from build123d import *

# Parameters (mm, degrees)
SKIZZE1_W                                            = 38
SKIZZE1_H                                            = 30
AUFSATZ_LINEAR_AUSTRAGEN1_DEPTH                      = 5
FORMSENKUNG_F_R_M4_SENKSCHRAUBE_MIT_SCHL_D           = 4.5
FORMSENKUNG_F_R_M4_SENKSCHRAUBE_MIT_SCHL_CSINK_D     = 9.4
FORMSENKUNG_F_R_M4_SENKSCHRAUBE_MIT_SCHL_CSINK_ANGLE = 90
F_8_0_8_DURCHMESSER_BOHRUNG1_D                       = 8


with BuildPart() as part:
    # Skizze1 → Aufsatz-Linear austragen1 (new body)
    with BuildSketch(Plane(origin=(0, 0, 0), x_dir=(1, 0, 0), z_dir=(0, 1, 0))):
        Rectangle(SKIZZE1_W, SKIZZE1_H)
    extrude(amount=AUFSATZ_LINEAR_AUSTRAGEN1_DEPTH)

    # Formsenkung für M4 Senkschraube mit Schlitz/Kreuzschlitz1 (through all)
    with Locations(Plane(origin=(0, 5, 0), x_dir=(1, 0, 0), z_dir=(0, 1, 0))):
        with Locations((-13, 8), (3, 8), (3, -8), (-13, -8), (13.76, 8), (13.76, -8)):
            CounterSinkHole(FORMSENKUNG_F_R_M4_SENKSCHRAUBE_MIT_SCHL_D / 2, FORMSENKUNG_F_R_M4_SENKSCHRAUBE_MIT_SCHL_CSINK_D / 2, counter_sink_angle=FORMSENKUNG_F_R_M4_SENKSCHRAUBE_MIT_SCHL_CSINK_ANGLE)

    # Ø8.0 (8) Durchmesser Bohrung1 (through all)
    with Locations(Plane(origin=(0, 5, 0), x_dir=(1, 0, 0), z_dir=(0, 1, 0))):
        with Locations((-5, 0)):
            Hole(F_8_0_8_DURCHMESSER_BOHRUNG1_D / 2)


solid = part.part
Design review of the part built by this model. Coordinates are the model's own, in mm. Coordinates: 2 decimals unless noted, no trailing zeros. Order: outer loops, then holes, each group sorted by start corner. A loop starts at its lowest first (then second) coordinate and runs counter-clockwise, first axis right, second up.
Item 1: For pin 1 Ø5 at (x, z) = (-13, -8) entering from +Y, flat-tipped, find the tip position at first contact; note if it passes through.
Item 2: Take a section at C-C, the plane y = 1.5. Write out the cut boundary in (x, z).
Item 3: Take a section at B-B, the plane z = 0. Write out the cut boundary in (x, y).
Item 4: For line 1 (Z direction, x = 3, y = 2.4); line 2 (X direction, y = 1.95, z = 8); line 3 (Z direction, x = 15, y = 0.9), list the stretches that pass through material, from the lowest coordinate up.
Item 5: Take a section at A-A, the plane x = 3. Write out the cut boundary in (y, z).
Item 6: Take a section at D-D, the plane x = -5. Write out the cut boundary in (y, z), then the cut area to 3 significant figures.
The answers:
1. pin 1: stops at y = 2.8
2. outline: (-19, -15) - (19, -15) - (19, 15) - (-19, 15) - close; hole circle Ø4.5 at (-13, -8); hole circle Ø4.5 at (-13, 8); hole circle Ø8 at (-5, 0); hole circle Ø4.5 at (3, -8); hole circle Ø4.5 at (3, 8); hole circle Ø4.5 at (13.76, -8); hole circle Ø4.5 at (13.76, 8)
3. outline: (-19, 0) - (-9, 0) - (-9, 5) - (-19, 5) - close; (-1, 0) - (19, 0) - (19, 5) - (-1, 5) - close
4. line 1: z = -15 to -10.25, -5.75 to 5.75, 10.25 to 15
4. line 2: x = -19 to -15.25, -10.75 to 0.75, 5.25 to 11.51, 16.01 to 19
4. line 3: z = -15 to -9.88, -6.12 to 6.12, 9.88 to 15
5. outline: (0, -15) - (5, -15) - (5, -12.7) - (2.55, -10.25) - (0, -10.25) - close; (0, -5.75) - (2.55, -5.75) - (5, -3.3) - (5, 3.3) - (2.55, 5.75) - (0, 5.75) - close; (0, 10.25) - (2.55, 10.25) - (5, 12.7) - (5, 15) - (0, 15) - close
6. outline: (0, -15) - (5, -15) - (5, -4) - (0, -4) - close; (0, 4) - (5, 4) - (5, 15) - (0, 15) - close
6. area: 110 mm2
